from build123d import *

# Parameters (mm, degrees)
F0_W     = 4
F0_H     = 47
F1_DEPTH = 21
F2_SIZE2 = 20.99999
F2_SIZE  = 19.99999


# Not quite as in the source:
# - a fillet or chamfer is up to 0.001 mm smaller than in the source, because OpenCascade refuses the exact size


with BuildPart() as f1:
    # F0 (on Front) → F1 (new body)
    with BuildSketch(Plane.XZ):
        Rectangle(F0_W, F0_H)
    extrude(amount=F1_DEPTH)

    # F2 (size 20 and 21 in the source; OpenCascade refuses exactly that, so slightly less here)
    f2_edges = [f1.edges().sort_by_distance(p)[0] for p in [
        (0, -21, 23.5),
    ]]
    f2_side = f1.faces().sort_by_distance((0, -21, 0))[0]
    chamfer(f2_edges, length=F2_SIZE, length2=F2_SIZE2, reference=f2_side)


solid = f1.part
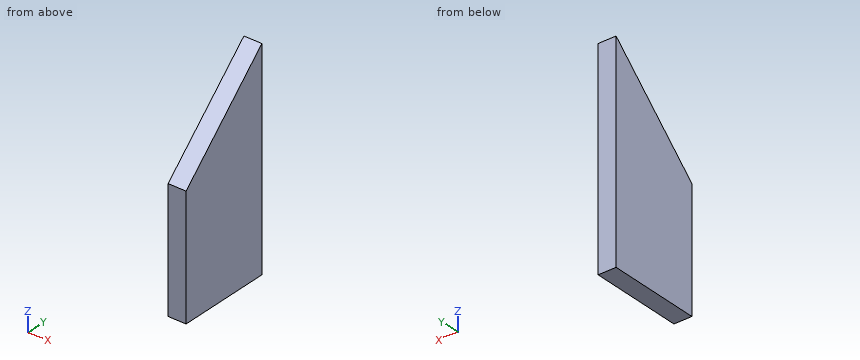
Could you check a few things on this model? Use its own coordinates, in mm. Round coordinates to 2 decimals unless told otherwise and drop trailing zeros. Write each loop counter-clockwise with the first axis right and the second up, starting at its lowest first coordinate (ties: lowest second). Pieces come first, ordered by that corner, then holes. Notation, with made-up numbers: (85.5, 79.5) - (92.5, 79.5) arc R17 cw to (92.5, 87.5) - close; hole circle Ø4 at (77.5, 56). An arc over 180 degrees is marked (long way). Put each result on its own line as item: value. Start each with the question number.
(1) I want a section at C-C, the plane y = -1.75. Please give me the cut outline in (x, z).
(2) Will this pin go through, and if not, where does the flat tip stop? pin 1 (1 mm diameter, centred on x = 1, y = -13.5, fed in from +Z).
(3) I want a section at B-B, the plane y = -6. Please give me the cut outline in (x, z), plus the area to 3 significant figures.
(4) I need wall thicknesses on probe 1 along Z at (x, y) = (-1.5, -18.75); probe 2 along Z at (x, y) = (1, -2); probe 3 along Y at (x, z) = (-0.35, 21.5). Which ranges of each line are inside material? Lowest first, please.
Here are the results:
1. outline: (-2, -23.5) - (2, -23.5) - (2, 21.83) - (-2, 21.83) - close
2. pin 1: stops at z = 11.12
3. outline: (-2, -23.5) - (2, -23.5) - (2, 17.79) - (-2, 17.79) - close
3. area: 165 mm^2
4. probe 1: z = -23.5 to 5.64
4. probe 2: z = -23.5 to 21.6
4. probe 3: y = -2.1 to 0
